from build123d import *

# Parameters (mm, degrees)
SKETCH029_W     = 110
SKETCH029_H     = 150
SKETCH029_R     = 2
SKETCH029_R_2   = 0.975
SKETCH029_R_3   = 1.5
PAD018_DEPTH    = 3
PAD019_DEPTH    = 57
SKETCH031_R     = 1.525
PAD020_DEPTH    = 5
POCKET007_DEPTH = 3


with BuildPart() as part:
    # Sketch029 → Pad018 (new body)
    with BuildSketch(Plane.XZ):
        with Locations((6.7, 54)):
            Rectangle(SKETCH029_W, SKETCH029_H)
        with Locations((-44.3, 100.2)):
            Circle(SKETCH029_R, mode=Mode.SUBTRACT)
        with Locations((-44.3, 7.8)):
            Circle(SKETCH029_R, mode=Mode.SUBTRACT)
        with Locations((56.7, 98)):
            Circle(SKETCH029_R_2, mode=Mode.SUBTRACT)
        with Locations((46.5, 120)):
            Circle(SKETCH029_R_2, mode=Mode.SUBTRACT)
        with Locations((-38.3, 74)):
            Circle(SKETCH029_R_3, mode=Mode.SUBTRACT)
        with Locations((1.7, 34)):
            Circle(SKETCH029_R_3, mode=Mode.SUBTRACT)
    extrude(amount=PAD018_DEPTH)

    # Sketch030 (on Face12 of Pad018) → Pad019 (join)
    with BuildSketch(Plane.XZ.offset(3)):
        Polygon((61.7, 129), (-48.3, 129), (-48.3, 105), (-45.3, 105), (-45.3, 126), (41.7, 126), (41.7, -18), (-45.3, -18), (-45.3, 3), (-48.3, 3), (-48.3, -21), (61.7, -21), (61.7, -18), (44.7, -18), (44.7, 126), (61.7, 126), align=None)
    extrude(amount=PAD019_DEPTH)

    # Sketch031 (on Face19 of Pad019) → Pad020 (join)
    with BuildSketch(Plane.XZ.offset(60)):
        Polygon((-48.3, -21), (-48.3, -6), (-33.3, -21), align=None)
        with Locations((-43.3, -16)):
            Circle(SKETCH031_R, mode=Mode.SUBTRACT)
        Polygon((-48.3, 129), (-48.3, 114), (-33.3, 129), align=None)
        with Locations((-43.3, 124)):
            Circle(SKETCH031_R, mode=Mode.SUBTRACT)
        Polygon((41.7, -21), (41.7, -6), (26.7, -21), align=None)
        with Locations((36.7, -16)):
            Circle(SKETCH031_R, mode=Mode.SUBTRACT)
        Polygon((41.7, 129), (41.7, 114), (26.7, 129), align=None)
        with Locations((36.7, 124)):
            Circle(SKETCH031_R, mode=Mode.SUBTRACT)
    extrude(amount=-PAD020_DEPTH)

    # Sketch032 (on Face37 of Pad020) → Pocket007 (cut)
    with BuildSketch(Plane(origin=(44.7, 0, 0), x_dir=(0, 0, 1), z_dir=(1, 0, 0))):
        with BuildLine():
            Line((126, 3), (126, 14))
            Line((126, 14), (66, 14))
            ThreePointArc((66, 14), (62.464466, 12.535534), (61, 9))
            Line((61, 9), (61, 3))
            Line((61, 3), (126, 3))
        make_face()
    extrude(amount=-POCKET007_DEPTH, mode=Mode.SUBTRACT)


solid = part.part
Build history of the part. All positions in model axes, mm. A direction names the side the tool comes from. Coordinates: 2 decimals unless noted, no trailing zeros. Write each loop counter-clockwise with the first axis right and the second up, starting at its lowest first coordinate (ties: lowest second). Pieces come first, ordered by that corner, then holes. Notation, with made-up numbers: (8, 88.25) -> (47, 88.25) arc R25 cw to (47, 101.25) -> close; hole circle Ø8 at (4, 86.5). An arc over 180 degrees is marked (long way). Use CSV: the item, a comma, the result in double quotes. Start each with the question number.
Q1. Cut at C-C, the plane x = -34.5. List the corners of the cut face in (y, z).
Q2. Flat gauge pins, fed straight in: pin 1 Ø5 at (x, z) = (14.5, 18.5) entering from -Y; pin 2 Ø2 at (y, z) = (-35, 15) entering from -X; pin 3 Ø1.2 at (x, z) = (56.7, 98) entering from +Y; pin 4 Ø6 at (y, z) = (-12, 63) entering from +X. Where does each tip first touch, or does it go through?
Q3. Drill centre lines: probe 1 along Z at (x, y) = (-44, -1); probe 2 along Z at (x, y) = (-36, -47.5); probe 3 along Z at (x, y) = (-38.3, -2.3). Where is each one in solid material? Low to high.
Q4. Cut at D-D, the plane y = -24.5. List the corners of the cut face in (x, z), then the cut area to 3 significant figures.
Q5. Pull direction Y, two halves, no side cores. Call faces 4 (the flat face through (6, 0, 55)), 5 (the flat face through (-42, -55, -14)), 6 (the cylindrical face through (-44.56, -1.479, 102.183)), 7 (the flat face through (-1, -31, -18)): released by +Y, released by -Y, zero draft, split by the parting line, or undercut.
Q6. Cut at B-B, the plane z = -12. List the corners of the cut face in (x, y).
Q7. 3-axis set-ups, long thin cutter, end or side, ignore diameter. For faces 1 (the flat face through (53, -31, -18)), 2 (the cylindrical face through (43, -13, 63)), 3 (the flat face through (-40.9, -57.5, -13.4)): which of +Z, -Z, +X, -X, +Y, -Y reach the whole face in a straight line?
Q8. Cut at A-A, the plane z = 84. List the corners of the cut face in (x, y), then the cut area to 3 significant figures.
Checked values:
1,outline,"(-60, -21) -> (0, -21) -> (0, 129) -> (-60, 129) -> (-60, 126) -> (-3, 126) -> (-3, -18) -> (-60, -18) -> close"
2,pin 1,"stops at y = -3"
2,pin 2,"stops at x = 41.7"
2,pin 3,"passes through"
2,pin 4,"stops at x = 44.7"
3,probe 1,"z = -21 to 5.82, 9.78 to 98.22, 102.18 to 129"
3,probe 2,"z = -21 to -18, 126 to 129"
3,probe 3,"z = -21 to 72.5, 75.5 to 129"
4,outline,"(-48.3, -21) -> (61.7, -21) -> (61.7, -18) -> (44.7, -18) -> (44.7, 126) -> (61.7, 126) -> (61.7, 129) -> (-48.3, 129) -> (-48.3, 105) -> (-45.3, 105) -> (-45.3, 126) -> (41.7, 126) -> (41.7, -18) -> (-45.3, -18) -> (-45.3, 3) -> (-48.3, 3) -> close"
4,area,"1,220 mm²"
5,face 4,"released by +Y"
5,face 5,"undercut"
5,face 6,"zero draft"
5,face 7,"undercut"
6,outline,"(-48.3, -60) -> (-42.3, -60) -> (-42.3, -55) -> (-45.3, -55) -> (-45.3, -3) -> (41.7, -3) -> (41.7, -55) -> (35.7, -55) -> (35.7, -60) -> (44.7, -60) -> (44.7, -3) -> (61.7, -3) -> (61.7, 0) -> (-48.3, 0) -> close"
7,face 1,"+X, -Y"
7,face 2,"+X, -X"
7,face 3,"-Y"
8,outline,"(-48.3, -3) -> (61.7, -3) -> (61.7, 0) -> (-48.3, 0) -> close; (41.7, -60) -> (44.7, -60) -> (44.7, -14) -> (41.7, -14) -> close"
8,area,"468 mm²"
